Here's how the part is built. I have some questions about the finished solid (model axes, mm). Face numbers are marked on the shaded views. Round coordinates to 2 decimals unless told otherwise and drop trailing zeros. Write each loop counter-clockwise with the first axis right and the second up, starting at its lowest first coordinate (ties: lowest second). Pieces come first, ordered by that corner, then holes. Notation, with made-up numbers: (-9, 12) -> (11, 12) arc R28 ccw to (11, 31) -> close; hole circle Ø2 at (48.25, 85.25). An arc over 180 degrees is marked (long way). Put each result on its own line as item: value. Start each with the question number.
1. We'd pull the mould along X, two halves only. Please class the marked faces 1, 2 and 3: +X half, -X half, draft (parallel to the pull), parting line (faces both ways), or undercut.
2. For pin 1 (3 mm diameter, centred on x = 0, z = 0, fed in from +Y), with a flat end and sliding along its axis, tell me the tip position at first contact or that it passes through.
3. Suppose I cut it at A-A (z = 0). Please give me the cut outline in (x, y).
4. Suppose I cut it at C-C (x = 0). Please give me the cut outline in (y, z), then the cut area to 3 significant figures.
5. Suppose I cut it at B-B (y = 2.65). Please give me the cut outline in (x, z), then the cut area to 3 significant figures.
6. Suppose I cut it at D-D (y = 0.6). Please give me the cut outline in (x, z), then the cut area to 3 significant figures.
7. I need wall thicknesses on probe 1 along X at (y, z) = (4.6, 0.4); probe 2 along Y at (x, z) = (10, 0.7); probe 3 along X at (y, z) = (2.15, 0). Which ranges of each line are inside material? Lowest first, please. Write a range as from..to.
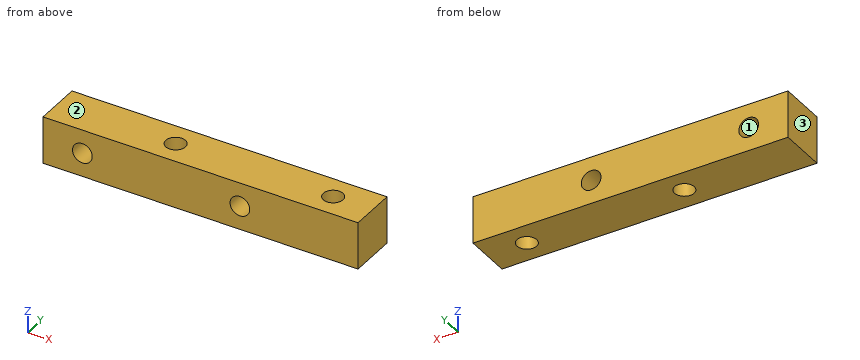
```python
from build123d import *

# Parameters (mm, degrees)
SKETCH1_W           = 40
SKETCH1_H           = 6
SKETCH1_R           = 1.25
BOSS_EXTRUDE1_DEPTH = 6
SKETCH2_R           = 1.25
CUT_EXTRUDE1_DEPTH  = 6


with BuildPart() as part:
    # Sketch1 → Boss-Extrude1 (new body)
    with BuildSketch(Plane(origin=(0, 0, 0), x_dir=(1, 0, 0), z_dir=(0, 1, 0))):
        with Locations((15, 0)):
            Rectangle(SKETCH1_W, SKETCH1_H)
        Circle(SKETCH1_R, mode=Mode.SUBTRACT)
        with Locations((20, 0)):
            Circle(SKETCH1_R, mode=Mode.SUBTRACT)
    extrude(amount=BOSS_EXTRUDE1_DEPTH)

    # Sketch2 → Cut-Extrude1 (cut)
    with BuildSketch(Plane.XY.offset(3)):
        with Locations((10, 3)):
            Circle(SKETCH2_R)
        with Locations((30, 3)):
            Circle(SKETCH2_R)
    extrude(amount=-CUT_EXTRUDE1_DEPTH, mode=Mode.SUBTRACT)


solid = part.part
```
Verdict:
1. face 1: undercut
1. face 2: draft
1. face 3: -X half
2. pin 1: stops at y = 6
3. outline: (-5, 0) -> (-1.25, 0) -> (-1.25, 6) -> (-5, 6) -> close; (1.25, 0) -> (18.75, 0) -> (18.75, 6) -> (1.25, 6) -> close; (21.25, 0) -> (35, 0) -> (35, 6) -> (21.25, 6) -> close; hole circle Ø2.5 at (10, 3); hole circle Ø2.5 at (30, 3)
4. outline: (0, -3) -> (6, -3) -> (6, -1.25) -> (0, -1.25) -> close; (0, 1.25) -> (6, 1.25) -> (6, 3) -> (0, 3) -> close
4. area: 21.0 mm^2
5. outline: (-5, -3) -> (8.8, -3) -> (8.8, 3) -> (-5, 3) -> close; (11.2, -3) -> (28.8, -3) -> (28.8, 3) -> (11.2, 3) -> close; (31.2, -3) -> (35, -3) -> (35, 3) -> (31.2, 3) -> close; hole circle Ø2.5 at (0, 0); hole circle Ø2.5 at (20, 0)
5. area: 201 mm^2
6. outline: (-5, -3) -> (35, -3) -> (35, 3) -> (-5, 3) -> close; hole circle Ø2.5 at (0, 0); hole circle Ø2.5 at (20, 0)
6. area: 230 mm^2
7. probe 1: x = -5..-1.18, 1.18..18.82, 21.18..35
7. probe 2: y = 0..1.75, 4.25..6
7. probe 3: x = -5..-1.25, 1.25..9.08, 10.92..18.75, 21.25..29.08, 30.92..35
